Geometry: final body of the model. Coordinates: model frame, mm. A direction names the side the tool comes from. Give positions to 0.01 mm unless a question says otherwise; leave off trailing zeros. Loops run counter-clockwise (first coordinate to the right, second up) from the corner with the lowest first, then second, coordinate; pieces in that order, holes last.
from build123d import *

# Parameters (mm, degrees)
SKETCH4_W           = 31.05
SKETCH4_H           = 18.45
BOSS_EXTRUDE1_DEPTH = 19
SHELL1_T            = 2
SKETCH5_W           = 12
SKETCH5_H           = 18.45
CUT_EXTRUDE1_DEPTH  = 2


with BuildPart() as part:
    # Sketch4 → Boss-Extrude1 (new body)
    with BuildSketch(Plane(origin=(0, 0, 0), x_dir=(0, 0, -1), z_dir=(1, 0, 0))):
        Rectangle(SKETCH4_W, SKETCH4_H)
    extrude(amount=BOSS_EXTRUDE1_DEPTH)

    # Shell1
    shell1_openings = [part.faces().sort_by_distance(p)[0] for p in [
        (0, 0, 0),
    ]]
    offset(amount=SHELL1_T, openings=shell1_openings, kind=Kind.INTERSECTION)

    # Sketch5 → Cut-Extrude1 (cut)
    with BuildSketch(Plane(origin=(0, 0, -17.525), x_dir=(-1, 0, 0), z_dir=(0, 0, -1))):
        with Locations((-6, 0)):
            Rectangle(SKETCH5_W, SKETCH5_H)
    extrude(amount=-CUT_EXTRUDE1_DEPTH, mode=Mode.SUBTRACT)


solid = part.part
Item 1: Pin query (flat end, axial travel): pin 1 (12 mm diameter, centred on y = -3, z = -11, fed in from -X); pin 2 (1 mm diameter, centred on y = -2, z = 4, fed in from -X); pin 3 (8 mm diameter, centred on x = 4.5, y = -3, fed in from -Z) (3 decimals). Return the tip coordinate at first contact, or that it passes through.
Values follow:
pin 1: stops at x = 12
pin 2: stops at x = 19
pin 3: stops at z = 15.525
Item 2: Section query B-B on y = 7.5. Return loops of the section in (x, z) (3 decimals).
Values follow:
outline: (0, 15.525) - (19, 15.525) - (19, -15.525) - (12, -15.525) - (12, -17.525) - (21, -17.525) - (21, 17.525) - (0, 17.525) - close
Item 3: Ray query, probe 1 along Z at (x, y) = (12.75, -3) (3 decimals); probe 2 along Y at (x, z) = (10.5, 4) (3 decimals); probe 3 along Z at (x, y) = (3.5, 8) (3 decimals). Return the intervals inside material, ascending.
Values follow:
probe 1: z = -17.525 to -15.525, 15.525 to 17.525
probe 2: y = -11.225 to -9.225, 9.225 to 11.225
probe 3: z = 15.525 to 17.525
Item 4: Draft query along Z for faces 1 (the face through (12, 0, -17)), 2 (the face through (10, 0, 17.525)), 3 (the face through (15, 0, -15.525)). Return one class per face: +Z half, -Z half, draft (parallel to the pull), parting line (faces both ways), or undercut.
Values follow:
face 1: draft
face 2: +Z half
face 3: undercut
Item 5: Section query C-C on x = 5.25. Return loops of the section in (y, z) (3 decimals).
Values follow:
outline: (-11.225, -17.525) - (-9.225, -17.525) - (-9.225, 15.525) - (9.225, 15.525) - (9.225, -17.525) - (11.225, -17.525) - (11.225, 17.525) - (-11.225, 17.525) - close
Item 6: Set-up query: faces 4 (the face through (9, -9.225, -1)), 5 (the face through (21, 0, 0)). Return all of +Z, -Z, +X, -X, +Y, -Y with unobstructed straight access to the full face (end or side cutting, diameter ignored); none if empty.
Values follow:
face 4: -X
face 5: +Z, -Z, +X, +Y, -Y
Item 7: Section query A-A on x = 15. Return loops of the section in (y, z) (3 decimals), plus the area to 3 significant figures.
Values follow:
outline: (-11.225, -17.525) - (11.225, -17.525) - (11.225, 17.525) - (-11.225, 17.525) - close; hole (-9.225, -15.525) - (9.225, -15.525) - (9.225, 15.525) - (-9.225, 15.525) - close
area: 214 mm2
